```python
from build123d import *

# Parameters (mm, degrees)
SKETCH_1_W             = 109
SKETCH_1_H             = 104
SM_BASE_FLANGE_1_DEPTH = 6
OTHER_START            = -52
OTHER_1_DEPTH          = 104
OTHER_1_2_DEPTH        = 104
CUT_EXTRUDE_1_DEPTH    = 108.693293005
CUT_EXTRUDE_2_REACH    = 127.065
SKETCH_8_R             = 6.5
CHAMFER_1_SIZE         = 0.5
CHAMFER_2_SIZE         = 5
FILLET_1_R             = 10
M6X1_01_D              = 5
M6X1_01_CSINK_D        = 6.5
M6X1_01_CSINK_ANGLE    = 90
M6X1_02_AT_2_COUNT     = 2
M6X1_02_AT_2_PITCH     = 47.376154339
M6X1_02_AT_3_COUNT     = 2
M6X1_02_AT_3_PITCH     = 47.376154339
M6X1_02_AT_4_COUNT     = 2
M6X1_02_AT_4_PITCH     = 64.717030361
SKETCH_9_R             = 12.5
SKETCH_9_R_2           = 3
CUT_EXTRUDE_3_DEPTH    = 6
CHAMFER_3_SIZE         = 1


# Read off the part's stored shape, not the designer's step: Изгиб1
# Sheet-metal steps are written as plain solids
with BuildPart() as part:
    # Sketch 1 → Базовая кромка1 (new body)
    with BuildSketch(Plane(origin=(0, 0, 0), x_dir=(1, 0, 0), z_dir=(0, 1, 0))):
        with Locations((54.5, 0)):
            Rectangle(SKETCH_1_W, SKETCH_1_H)
    extrude(amount=-SM_BASE_FLANGE_1_DEPTH)

    # Other 1 outline → Other 1 (cut)
    with BuildSketch(Plane.XY.offset(OTHER_START)):
        with BuildLine():
            Line((109, 0), (51.507997892, 0))
            Line((51.507997892, 0), (51.106946786, -0.522660023))
            ThreePointArc((51.106946786, -0.522660023), (46.192041675, -4.556218407), (40, -6.000000028))
            Line((40, -6.000000028), (109, -6))
            Line((109, -6), (109, 0))
        make_face()
    extrude(amount=OTHER_1_DEPTH, mode=Mode.SUBTRACT)

    # Other 1 2 outline → Other 1 2 (add)
    with BuildSketch(Plane.XY.offset(OTHER_START)):
        with BuildLine():
            ThreePointArc((71.183364554, 26.500000037), (64.991322874, 25.056218415), (60.07641776, 21.022660029))
            Line((60.07641776, 21.022660029), (46.346826745, 3.129908551))
            ThreePointArc((46.346826745, 3.129908551), (43.538309534, 0.825018043), (40, -2.8e-08))
            Line((40, -2.8e-08), (51.507997892, 0))
            Line((51.507997892, 0), (64.836537802, 17.370091455))
            ThreePointArc((64.836537802, 17.370091455), (67.645055016, 19.674981966), (71.183364554, 20.500000037))
            Line((71.183364554, 20.500000037), (109, 20.5))
            Line((109, 20.5), (109, 26.5))
            Line((109, 26.5), (71.183364554, 26.500000037))
        make_face()
    extrude(amount=OTHER_1_2_DEPTH)

    # Эскиз5 → Вытянуть1 (cut, through all)
    with BuildSketch(Plane(origin=(27.659504319, -21.223884138, 0), x_dir=(0.608761429008719, 0.7933533402912364, 0), z_dir=(-0.7933533402912364, 0.608761429008719, 0))):
        Polygon((33.697283883, 52), (50.250603481, 27.5), (53.250603481, 27.5), (87.37885928, 27.5), (87.37885928, 52), align=None)
        Polygon((87.37885928, -52), (33.697283883, -52), (50.250603481, -27.5), (53.250603481, -27.5), (87.37885928, -27.5), align=None)
    extrude(amount=-CUT_EXTRUDE_1_DEPTH, mode=Mode.SUBTRACT)

    # Эскиз8 → Вытянуть2 (cut, up to next)
    with BuildSketch(Plane(origin=(0, 26.5, 0), x_dir=(1, 0, 0), z_dir=(0, 1, 0)), mode=Mode.PRIVATE) as cut_extrude_2_sk1:
        with Locations(Location((94, 12.5, 0), (0, 0, 270))):
            Circle(SKETCH_8_R)
    cut_extrude_2_tool1 = extrude(cut_extrude_2_sk1.sketch, amount=-CUT_EXTRUDE_2_REACH, mode=Mode.PRIVATE) & part.part
    # Эскиз8 → Вытянуть2 (cut, up to next)
    with BuildSketch(Plane(origin=(0, 26.5, 0), x_dir=(1, 0, 0), z_dir=(0, 1, 0)), mode=Mode.PRIVATE) as cut_extrude_2_sk2:
        with Locations(Location((94, -12.5, 0), (0, 0, 270))):
            Circle(SKETCH_8_R)
    cut_extrude_2_tool2 = extrude(cut_extrude_2_sk2.sketch, amount=-CUT_EXTRUDE_2_REACH, mode=Mode.PRIVATE) & part.part
    add(cut_extrude_2_tool1.solids().sort_by_distance((94, 26.5, -12.5))[0], mode=Mode.SUBTRACT)
    add(cut_extrude_2_tool2.solids().sort_by_distance((94, 26.5, 12.5))[0], mode=Mode.SUBTRACT)

    # Фаска1
    chamfer_1_edges = [part.edges().sort_by_distance(p)[0] for p in [
        (94, 26.5, -19),
        (94, 26.5, 6),
    ]]
    chamfer(chamfer_1_edges, length=CHAMFER_1_SIZE)

    # Фаска2
    chamfer_2_edges = [part.edges().sort_by_distance(p)[0] for p in [
        (109, 23.5, -27.5),
        (109, 23.5, 27.5),
    ]]
    chamfer(chamfer_2_edges, length=CHAMFER_2_SIZE)

    # Скругление1
    fillet_1_edges = [part.edges().sort_by_distance(p)[0] for p in [
        (50.553171029, 3.683684303, -52),
        (50.553171029, 3.683684303, 52),
    ]]
    fillet(fillet_1_edges, radius=FILLET_1_R)

    # Зеркальное отражение1: part across plane


with BuildPart() as part_1:
    add(part.part)
    add(part.part.mirror(Plane(origin=(0, -6, -52), x_dir=(0, 0, 1), z_dir=(-1, 0, 0))))

    # Отверстие обработанное метчиком M6x1.01 (through all)
    with Locations(Plane(origin=(29.011851027, 0, 16.75), x_dir=(0, 0, 1), z_dir=(0, 1, 0))):
        with Locations((0, 0), (12.261851027, -45.761851027), (-33.5, -58.023702054), (-33.5, 0)):
            CounterSinkHole(M6X1_01_D / 2, M6X1_01_CSINK_D / 2, counter_sink_angle=M6X1_01_CSINK_ANGLE)

    # Эскиз11 → Отверстие обработанное метчиком M6x1.02 (revolve, cut)
    with BuildSketch(Plane(origin=(-29.011851027, 0, 16.75), x_dir=(0, 0, 1), z_dir=(1, 0, 0))):
        Polygon((0, 0), (0, 6.000000028), (3.25, 6.000000028), (2.5, 5.250000028), (2.5, 0), align=None)
    m6x1_02 = revolve(axis=Axis((-29.011851027, 6.35, 16.75), (0, -1, 0)), mode=Mode.SUBTRACT)

    # Отверстие обработанное метчиком M6x1.02 at 2: Отверстие обработанное метчиком M6x1.02 ×2
    with Locations(*[Vector(0.9659258262890683, 0, 0.2588190451025209) * (i * M6X1_02_AT_2_PITCH) for i in range(1, M6X1_02_AT_2_COUNT)]):
        add(m6x1_02, mode=Mode.SUBTRACT)

    # Отверстие обработанное метчиком M6x1.02 at 3: Отверстие обработанное метчиком M6x1.02 ×2
    with Locations(*[Vector(0.25881904510252063, 0, -0.9659258262890683) * (i * M6X1_02_AT_3_PITCH) for i in range(1, M6X1_02_AT_3_COUNT)]):
        add(m6x1_02, mode=Mode.SUBTRACT)

    # Отверстие обработанное метчиком M6x1.02 at 4: Отверстие обработанное метчиком M6x1.02 ×2
    with Locations(*[Vector(0.7071067811865474, 0, -0.7071067811865478) * (i * M6X1_02_AT_4_PITCH) for i in range(1, M6X1_02_AT_4_COUNT)]):
        add(m6x1_02, mode=Mode.SUBTRACT)

    # Эскиз9 → Вытянуть3 (cut)
    with BuildSketch(Plane(origin=(0, 0, 0), x_dir=(1, 0, 0), z_dir=(0, 1, 0))):
        with Locations(Location((0, 0, 0), (0, 0, 270))):
            Circle(SKETCH_9_R)
        with Locations(Location((0, 33.5, 0), (0, 0, 270))):
            Circle(SKETCH_9_R_2)
        with Locations(Location((0, -33.5, 0), (0, 0, 270))):
            Circle(SKETCH_9_R_2)
        with Locations(Location((-33.5, 0, 0), (0, 0, 270))):
            Circle(SKETCH_9_R_2)
        with Locations(Location((33.5, 0, 0), (0, 0, 270))):
            Circle(SKETCH_9_R_2)
    extrude(amount=-CUT_EXTRUDE_3_DEPTH, mode=Mode.SUBTRACT)

    # Фаска3
    chamfer_3_edges = [part_1.edges().sort_by_distance(p)[0] for p in [
        (0, -6, -12.5),
    ]]
    chamfer(chamfer_3_edges, length=CHAMFER_3_SIZE)

    # Эскиз12 → Вырез-Повернуть1 (revolve, cut)
    with BuildSketch(Plane(origin=(0, 0, 0), x_dir=(1, 0, 0), z_dir=(0, 1, 0))):
        with BuildLine():
            Line((0, 46.5), (0, 45.5))
            ThreePointArc((0, 45.5), (0.5, 46), (0, 46.5))
        make_face()
    revolve(axis=Axis((0, 0, -52), (0, 0, 1)), mode=Mode.SUBTRACT)


solid = part_1.part
```
Could you check a few things on this model? Use its own coordinates, in mm. A direction names the side the tool comes from. Coordinates: 2 decimals unless noted, no trailing zeros. Loops run counter-clockwise (first coordinate to the right, second up) from the corner with the lowest first, then second, coordinate; pieces in that order, holes last. Notation, with made-up numbers: M 79.5,19 L 112.5,19 A18 ccw 112.5,29 Z; hole C 11,-9.5 d8. An arc over 180 degrees is marked long. Put each result on its own line as item: value. Start each with the question number.
(1) I need wall thicknesses on line 1 (Z direction, x = -16.75, y = -3.35); line 2 (X direction, y = -3, z = -16); line 3 (X direction, y = -4.7, z = 0). Which ranges of each line are inside material? Lowest first, please. Write a range as from..to.
(2) Suppose I cut it at A-A on x = -16.75. Please give me the cut outline in (y, z).
(3) Will these pins go through, and if not, where does the flat tip stop? P1, Ø10.5, axis at x = -94, z = -12.5, coming from the +Y side; P2, Ø8, axis at x = 68.5, z = 25.5, coming from the -Y side; P3, Ø6, axis at x = -29.01, z = 16.75, coming from the +Y side; P4, Ø6, axis at x = 78, y = 23, coming from the -Z side.
(4) Thinking about a two-plate mould opening in X: for faces 1 (the face through (-80, 23, -27.5)), 2 (the face through (67.599, 19.652, -0.385)), 3 (the face through (-87.655, 23.289, 11.091)), which applies, pulls with the +X half, pulls with the -X half, needs draft (parallel to the pull), parting line crosses it, or undercut?
(5) Suppose I cut it at B-B on x = -82.5. Please give me the cut outline in (y, z), then the cut area to 3 significant figures.
(6) Suppose I cut it at C-C on z = -16.75. Count the separate pieces of the cut face and the enclosed holes in it, then the cut area to 3 significant figures.
(7) For faces 4 (the face through (65.072, 25.096, -0.385)), 5 (the face through (-90, 20.5, 0)), 6 (the face through (-56.406, 11.38, -37.69)), which set-ups out of +Z, -Z, +X, -X, +Y, -Y let a thin tool reach every point of the face, with its end or its side?
Solutions:
1. line 1: z = -52..-31.51, -26.51..26.51, 31.51..52
1. line 2: x = -48.66..-31.4, -26.63..26.63, 31.4..48.66
1. line 3: x = -45.89..-36.5, -30.5..-12.5, 12.5..30.5, 36.5..45.89
2. outline: M -6,-52 L 0,-52 L 0,-31.51 L -5.25,-31.51 L -6,-32.26 Z; M -6,-25.76 L -5.25,-26.51 L 0,-26.51 L 0,25.76 L -0.75,26.51 L -6,26.51 Z; M -6,31.51 L -0.75,31.51 L 0,32.26 L 0,52 L -6,52 Z
3. P1: passes through
3. P2: stops at y = 16.93
3. P3: stops at y = 0
3. P4: stops at z = -27.5
4. face 1: needs draft
4. face 2: pulls with the +X half
4. face 3: undercut
5. outline: M 20.5,-27.5 L 26.5,-27.5 L 26.5,27.5 L 20.5,27.5 Z
5. area: 330 mm2
6. separate pieces: 5
6. enclosed holes: 0
6. area: 1,270 mm2
7. face 4: +Z, -Z, +Y
7. face 5: +Z, -Z, -X, -Y
7. face 6: -Z, -X, +Y
